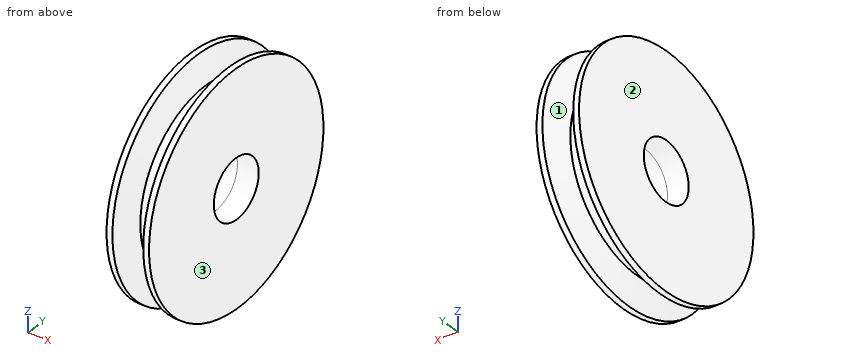
from build123d import *

# Parameters (mm, degrees)
F2_R     = 17.5
F3_DEPTH = 25


with BuildPart() as f1:
    # F0 (on Front) → F1 (revolve)
    with BuildSketch(Plane.XZ):
        Polygon((0, 37.8452404466), (0, 0), (12.7, 0), (12.7, 52.3875), (4.4460149232, 52.3875), align=None)
        Polygon((0, 52.3875), (0, 37.8452404466), (4.4460149232, 52.3875), align=None)
        Polygon((9.20242, 67.945), (4.4460149232, 52.3875), (12.7, 52.3875), (12.7, 67.945), align=None)
    revolve(axis=Axis((21.4788783342, 0, 0), (1, 0, 0)))

    # F2 (on face) → F3 (cut)
    with BuildSketch(Plane(origin=(0, 0, 0), x_dir=(0, -1, 0), z_dir=(-1, 0, 0))):
        Circle(F2_R)
    extrude(amount=-F3_DEPTH, mode=Mode.SUBTRACT)

    # F4: F1 across plane


with BuildPart() as f1_1:
    add(f1.part)
    add(f1.part.mirror(Plane.YZ))


solid = f1_1.part
Here's how the part is built. I have some questions about the finished solid (model axes, mm). Face numbers are marked on the shaded views. Give positions to 0.01 mm unless a question says otherwise; leave off trailing zeros. Order: outer loops, then holes, each group sorted by start corner. A loop starts at its lowest first (then second) coordinate and runs counter-clockwise, first axis right, second up. Notation, with made-up numbers: M 41,72 L 77,72 A20 ccw 77,92 Z; hole C 88.5,77.25 d10. An arc over 180 degrees is marked long. Answer as a JSON object with one key per item and string values. Group by question number.
1) We'd pull the mould along X, two halves only. Please class the marked faces 1, 2 and 3: pulls with the +X half, pulls with the -X half, needs draft (parallel to the pull), parting line crosses it, or undercut.
2) Please list where these lines run through material, in increasing order: L1, parallel to Z at x = 3, y = 0; L2, parallel to Z at x = -10, y = 0 (3 decimals); L3, parallel to X at y = -15, z = -62. Write a range as [from, to].
3) I'm going to push flat-ended pins straight in: pin 1 Ø1 at (x, z) = (-1, 43.5) entering from +Y; pin 2 Ø3 at (x, z) = (1.5, -38.5) entering from +Y; pin 3 Ø12 at (y, z) = (-9.5, -1.5) entering from +X (3 decimals); pin 4 Ø10 at (x, y) = (-7, 0) entering from -Z (3 decimals). Where does each tip first touch, or does it pass through?
4) Suppose I cut it at A-A, the plane y = 0. Write out the boundary of the cut face in (x, z) (1 decimal).
Results found:
{
 "1": {"face 1": "undercut", "face 2": "pulls with the -X half", "face 3": "pulls with the +X half"},
 "2": {"L1": "[-52.39, -17.5], [17.5, 52.39]", "L2": "[-67.945, -17.5], [17.5, 67.945]", "L3": "[-12.7, -7.93], [7.93, 12.7]"},
 "3": {"pin 1": "y = 29.92", "pin 2": "y = 37.09", "pin 3": "through", "pin 4": "z = -67.945"},
 "4": {"outline": "M -12.7,-67.9 L -9.2,-67.9 L -4.4,-52.4 L 4.4,-52.4 L 9.2,-67.9 L 12.7,-67.9 L 12.7,-17.5 L -12.7,-17.5 Z; M -12.7,17.5 L 12.7,17.5 L 12.7,67.9 L 9.2,67.9 L 4.4,52.4 L -4.4,52.4 L -9.2,67.9 L -12.7,67.9 Z"}
}
